```python
from build123d import *

# Parameters (mm, degrees)
SKETCH1_W           = 80
SKETCH1_H           = 100
BOSS_EXTRUDE1_DEPTH = 3.175
CUT_EXTRUDE2_REACH  = 5.175
SKETCH4_W           = 80
SKETCH4_H           = 3.175
BOSS_EXTRUDE2_DEPTH = 60
SKETCH5_R           = 3.175
CUT_EXTRUDE3_DEPTH  = 3.175
SKETCH6_W           = 80
SKETCH6_H           = 10
CUT_EXTRUDE4_DEPTH  = 64.175


with BuildPart() as part:
    # Sketch1 → Boss-Extrude1 (new body)
    with BuildSketch(Plane.XY):
        with Locations((40, -50)):
            Rectangle(SKETCH1_W, SKETCH1_H)
        with BuildLine():
            Line((18.98, -16.93), (18.98, -35.93))
            ThreePointArc((18.98, -35.93), (16.43, -38.48), (13.88, -35.93))
            Line((13.88, -35.93), (13.88, -16.93))
            ThreePointArc((13.88, -16.93), (16.43, -14.38), (18.98, -16.93))
        make_face(mode=Mode.SUBTRACT)
        with BuildLine():
            Line((61.02, -16.93), (61.02, -35.93))
            ThreePointArc((61.02, -35.93), (63.57, -38.48), (66.12, -35.93))
            Line((66.12, -35.93), (66.12, -16.93))
            ThreePointArc((66.12, -16.93), (63.57, -14.38), (61.02, -16.93))
        make_face(mode=Mode.SUBTRACT)
        with BuildLine():
            Line((18.98, -83.07), (18.98, -64.07))
            ThreePointArc((18.98, -64.07), (16.43, -61.52), (13.88, -64.07))
            Line((13.88, -64.07), (13.88, -83.07))
            ThreePointArc((13.88, -83.07), (16.43, -85.62), (18.98, -83.07))
        make_face(mode=Mode.SUBTRACT)
        with BuildLine():
            Line((61.02, -83.07), (61.02, -64.07))
            ThreePointArc((61.02, -64.07), (63.57, -61.52), (66.12, -64.07))
            Line((66.12, -64.07), (66.12, -83.07))
            ThreePointArc((66.12, -83.07), (63.57, -85.62), (61.02, -83.07))
        make_face(mode=Mode.SUBTRACT)
    extrude(amount=BOSS_EXTRUDE1_DEPTH)

    # Sketch2 → Cut-Extrude2 (cut, up to next)
    with BuildSketch(Plane.XY.offset(3.175), mode=Mode.PRIVATE) as cut_extrude2_sk1:
        with BuildLine():
            Line((25, -35), (25, -100))
            Line((25, -100), (55, -100))
            Line((55, -100), (55, -35))
            ThreePointArc((55, -35), (40, -20), (25, -35))
        make_face()
    cut_extrude2_tool1 = extrude(cut_extrude2_sk1.sketch, amount=-CUT_EXTRUDE2_REACH, mode=Mode.PRIVATE) & part.part
    add(cut_extrude2_tool1.solids().sort_by_distance((40, -61.536522, 3.175))[0], mode=Mode.SUBTRACT)

    # Sketch4 → Boss-Extrude2 (add)
    with BuildSketch(Plane(origin=(0, 0, 0), x_dir=(-1, 0, 0), z_dir=(0, 0, -1))):
        with Locations((-40, -1.5875)):
            Rectangle(SKETCH4_W, SKETCH4_H)
    extrude(amount=BOSS_EXTRUDE2_DEPTH)

    # Sketch5 → Cut-Extrude3 (cut)
    with BuildSketch(Plane(origin=(0, 0, 0), x_dir=(1, 0, 0), z_dir=(0, 1, 0))):
        with Locations((7, 53.825)):
            Circle(SKETCH5_R)
        with Locations((7, 6.825)):
            Circle(SKETCH5_R)
        with Locations((72, 53.825)):
            Circle(SKETCH5_R)
        with Locations((72, 6.825)):
            Circle(SKETCH5_R)
    extrude(amount=-CUT_EXTRUDE3_DEPTH, mode=Mode.SUBTRACT)

    # Sketch6 → Cut-Extrude4 (cut, through all)
    with BuildSketch(Plane.XY.offset(3.175)):
        with Locations((40, -95)):
            Rectangle(SKETCH6_W, SKETCH6_H)
    extrude(amount=-CUT_EXTRUDE4_DEPTH, mode=Mode.SUBTRACT)


solid = part.part
```
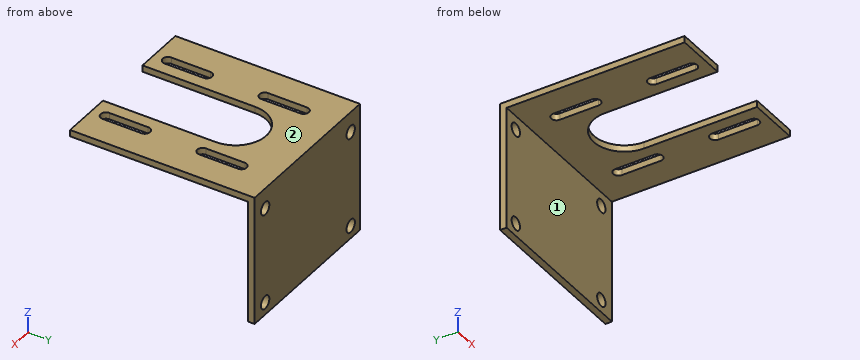
Input: part model. Units: mm. Frame: model coordinates. Face numbers are marked on the shaded views. A direction names the side the tool comes from. Give positions to 0.01 mm unless a question says otherwise; leave off trailing zeros. Write each loop counter-clockwise with the first axis right and the second up, starting at its lowest first coordinate (ties: lowest second). Pieces come first, ordered by that corner, then holes. Notation, with made-up numbers: (83.5, 31.5) - (120.5, 31.5) arc R21 cw to (120.5, 51.5) - close; hole circle Ø11 at (10, 34). An arc over 180 degrees is marked (long way). Write item = value, one per line. Start each with the question number.
1) Cut plane A-A (x = 63.57). Return loops of the section in (y, z) (3 decimals).
2) Cut plane D-D (x = 27). Return loops of the section in (y, z) (3 decimals), and give its area (3 significant figures).
3) Material intervals for L1, parallel to Z at x = 72, y = -0.95 (3 decimals); L2, parallel to X at y = -53, z = 0.5; L3, parallel to Z at x = 68, y = -50 (3 decimals), sorted ascending. Write a range as [from, to].
4) Pin query (flat end, axial travel): pin 1 (12 mm diameter, centred on x = 18.5, y = -11, fed in from -Z); pin 2 (18 mm diameter, centred on x = 37, z = -16.5, fed in from -Y) (3 decimals). Return the tip coordinate at first contact, or that it passes through.
5) Cut plane B-B (z = -52). Return loops of the section in (x, y) (3 decimals).
6) Cut plane C-C (y = -28.5). Return loops of the section in (x, z) (1 decimal).
7) Reachability of the marked faces 1 and 2 from +Z, -Z, +X, -X, +Y, -Y: full face, straight path, thin tool, end or side. Return the list, or none.
Answers follow:
q1.outline = (-90, 0) - (-85.62, 0) - (-85.62, 3.175) - (-90, 3.175) - close; (-61.52, 0) - (-38.48, 0) - (-38.48, 3.175) - (-61.52, 3.175) - close; (-14.38, 0) - (-3.175, 0) - (-3.175, -60) - (0, -60) - (0, 3.175) - (-14.38, 3.175) - close
q2.outline = (-27.517, 0) - (-3.175, 0) - (-3.175, -60) - (0, -60) - (0, 3.175) - (-27.517, 3.175) - close
q2.area = 278 mm^2
q3.L1 = [-60, -57], [-50.65, -10], [-3.65, 3.175]
q3.L2 = [0, 25], [55, 80]
q3.L3 = [0, 3.175]
q4.pin_1 = 0
q4.pin_2 = -3.175
q5.outline = (0, -3.175) - (4.402, -3.175) - (4.402, 0) - (0, 0) - close; (9.598, -3.175) - (69.402, -3.175) - (69.402, 0) - (9.598, 0) - close; (74.598, -3.175) - (80, -3.175) - (80, 0) - (74.598, 0) - close
q6.outline = (0, 0) - (13.9, 0) - (13.9, 3.2) - (0, 3.2) - close; (19, 0) - (26.5, 0) - (26.5, 3.2) - (19, 3.2) - close; (53.5, 0) - (61, 0) - (61, 3.2) - (53.5, 3.2) - close; (66.1, 0) - (80, 0) - (80, 3.2) - (66.1, 3.2) - close
q7.face_1 = -Z, +X, -X, -Y
q7.face_2 = +Z, +X, -X, +Y, -Y
